Can you work these out from the model? Positions are in its coordinate system, mm. Face numbers are marked on the shaded views. A direction names the side the tool comes from. Give positions to 0.01 mm unless a question says otherwise; leave off trailing zeros. Loops run counter-clockwise (first coordinate to the right, second up) from the corner with the lowest first, then second, coordinate; pieces in that order, holes last. Notation, with made-up numbers: (81.25, -20) - (132.25, -20) arc R19 cw to (132.25, 0) - close; hole circle Ø9 at (7.25, 57). An arc over 180 degrees is marked (long way). Answer as a JSON object with one key per item and string values.
```python
from build123d import *

# Parameters (mm, degrees)
F1_DEPTH = 10
F0_W     = 15
F0_H     = 15
F2_DEPTH = 25


with BuildPart() as f1:
    # F0 (on Front) → F1 (new body)
    with BuildSketch(Plane.XZ):
        Polygon((-48.808126, 51.012476), (-58.808126, 51.012476), (-58.808126, -23.987524), (-48.808126, -23.987524), (-48.808126, -8.987524), align=None)
    extrude(amount=F1_DEPTH)

    # F0 (on Front) → F2 (join)
    with BuildSketch(Plane.XZ):
        with Locations((-41.308126, -16.487524)):
            Rectangle(F0_W, F0_H)
    extrude(amount=F2_DEPTH)


solid = f1.part
```
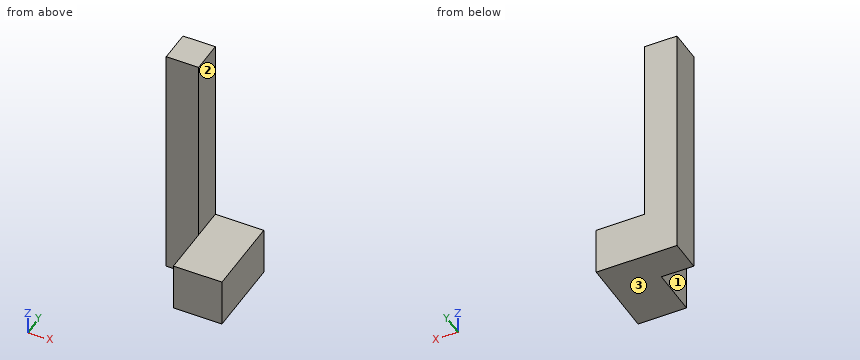
1) Imagine slicing it at A-A on z = -13. Write out the boundary of the cut face in (x, y).
Check sheet entries:
{"outline": "(-58.81, -10) - (-48.81, -10) - (-48.81, -25) - (-33.81, -25) - (-33.81, 0) - (-58.81, 0) - close"}
2) I'm going to push flat-ended pins straight in: P1, Ø7.5, axis at x = -43.5, y = -15, coming from the +Z side; P2, Ø11, axis at y = -5.5, z = 19.5, coming from the +X side; P3, Ø4.5, axis at y = -20.5, z = -16.5, coming from the -X side. Where does each tip first touch, or does it pass through?
Check sheet entries:
{"P1": "z = -8.99", "P2": "x = -48.81", "P3": "x = -48.81"}
3) Imagine slicing it at C-C on y = -20.25. Write out the boundary of the cut face in (x, z).
Check sheet entries:
{"outline": "(-48.81, -23.99) - (-33.81, -23.99) - (-33.81, -8.99) - (-48.81, -8.99) - close"}
4) I need wall thicknesses on L1, parallel to Z at x = -41.25, y = -6.75; L2, parallel to Y at x = -56, z = 4; L3, parallel to X at y = -1.25, z = 46.5. Which ranges of each line are inside material? Lowest first, please.
Check sheet entries:
{"L1": "-23.99 to -8.99", "L2": "-10 to 0", "L3": "-58.81 to -48.81"}
5) Imagine slicing it at D-D on y = -5. Write out the boundary of the cut face in (x, z).
Check sheet entries:
{"outline": "(-58.81, -23.99) - (-33.81, -23.99) - (-33.81, -8.99) - (-48.81, -8.99) - (-48.81, 51.01) - (-58.81, 51.01) - close"}
6) Which directions (+Z, -Z, +X, -X, +Y, -Y) give clear straight access to the entire face, cutting with the end or side of a thin tool? Please do the marked faces 1, 2 and 3.
Check sheet entries:
{"face 1": "+Z, -Z, -X, -Y", "face 2": "+Z, +X, +Y, -Y", "face 3": "-Z, +X, -X, +Y, -Y"}
7) Imagine slicing it at B-B on x = -46.75. Write out the boundary of the cut face in (y, z), and give its area (3 significant figures).
Check sheet entries:
{"outline": "(-25, -23.99) - (0, -23.99) - (0, -8.99) - (-25, -8.99) - close", "area": "375 mm2"}
